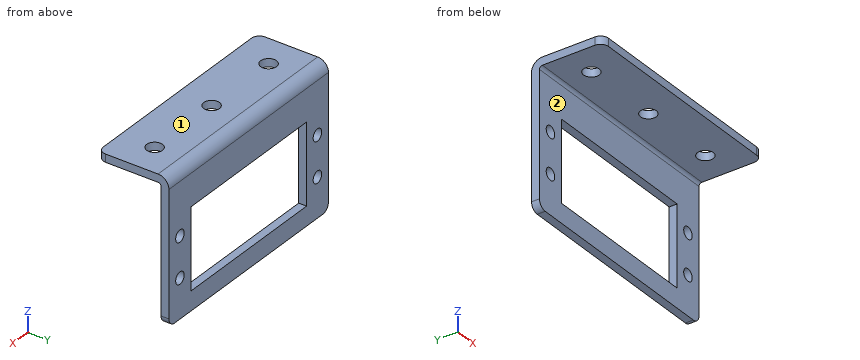
from build123d import *

# Parameters (mm, degrees)
SKETCH1_W                    = 56
SKETCH1_H                    = 34
BASE_FLANGE1_DEPTH           = 2
EDGE_FLANGE1_STRIP_W         = 9.4732
EDGE_FLANGE1_STRIP_H         = 2
EDGE_FLANGE1_STRIP_CUT_DEPTH = 56
EDGE_FLANGE1_DEPTH           = 56
SKETCH9_W                    = 40.64
SKETCH9_H                    = 20.32
CUT_EXTRUDE1_DEPTH           = 39.327535793
SKETCH10_R                   = 1.5
CUT_EXTRUDE2_DEPTH           = 39.327535793
FILLET1_R                    = 2
SKETCH11_R                   = 2
CUT_EXTRUDE3_DEPTH           = 48.581509013


# Sheet-metal steps are written as plain solids
with BuildPart() as part:
    # Sketch1 → Base-Flange1 (new body)
    with BuildSketch(Plane(origin=(0, 0, 0), x_dir=(1, 0, 0), z_dir=(0, 1, 0))):
        Rectangle(SKETCH1_W, SKETCH1_H)
    extrude(amount=-BASE_FLANGE1_DEPTH)

    # Edge-Flange1 strip (across the edge) → Edge-Flange1 strip cut (cut)
    with BuildSketch(Plane(origin=(28, -2, 17), x_dir=(0, 0, -1), z_dir=(-1, 0, 0))):
        with Locations((-4, -1)):
            Rectangle(EDGE_FLANGE1_STRIP_W, EDGE_FLANGE1_STRIP_H)
    extrude(amount=EDGE_FLANGE1_STRIP_CUT_DEPTH, mode=Mode.SUBTRACT)

    # Edge-Flange1 section (across the edge) → Edge-Flange1 (add)
    with BuildSketch(Plane(origin=(28, -2, 17), x_dir=(0, 0, -1), z_dir=(-1, 0, 0))):
        with BuildLine():
            Line((-2, 0.7366), (-2, 16))
            Line((-2, 16), (0, 16))
            Line((0, 16), (0, 0.7366))
            ThreePointArc((0, 0.7366), (0.215745145, 0.215745145), (0.7366, 0))
            Line((0.7366, 0), (0.7366, -2))
            ThreePointArc((0.7366, -2), (-1.198468417, -1.198468417), (-2, 0.7366))
        make_face()
    extrude(amount=EDGE_FLANGE1_DEPTH)

    # Sketch9 → Cut-Extrude1 (cut, through all)
    with BuildSketch(Plane(origin=(0, 0, 0), x_dir=(1, 0, 0), z_dir=(0, 1, 0))):
        with Locations((0, 2)):
            Rectangle(SKETCH9_W, SKETCH9_H)
    extrude(amount=-CUT_EXTRUDE1_DEPTH, mode=Mode.SUBTRACT)

    # Sketch10 → Cut-Extrude2 (cut, through all)
    with BuildSketch(Plane(origin=(0, 0, 0), x_dir=(1, 0, 0), z_dir=(0, 1, 0))):
        with Locations(Location((-24.13, 7.08, 0), (0, 0, 270))):
            Circle(SKETCH10_R)
        with Locations(Location((-24.13, -3.08, 0), (0, 0, 270))):
            Circle(SKETCH10_R)
        with Locations(Location((24.13, 7.08, 0), (0, 0, 270))):
            Circle(SKETCH10_R)
        with Locations(Location((24.13, -3.08, 0), (0, 0, 270))):
            Circle(SKETCH10_R)
    extrude(amount=-CUT_EXTRUDE2_DEPTH, mode=Mode.SUBTRACT)

    # Fillet1
    fillet1_edges = [part.edges().sort_by_distance(p)[0] for p in [
        (28, -18, 18),
        (-28, -18, 18),
        (-28, -1, -17),
        (28, -1, -17),
    ]]
    fillet(fillet1_edges, radius=FILLET1_R)

    # Sketch11 → Cut-Extrude3 (cut, through all)
    with BuildSketch(Plane(origin=(0, 0, 17), x_dir=(-1, 0, 0), z_dir=(0, 0, -1))):
        with Locations(Location((0, -9.3683, 0), (0, 0, 90))):
            Circle(SKETCH11_R)
        with Locations(Location((-20, -9.3683, 0), (0, 0, 90))):
            Circle(SKETCH11_R)
        with Locations(Location((20, -9.3683, 0), (0, 0, 90))):
            Circle(SKETCH11_R)
    extrude(amount=-CUT_EXTRUDE3_DEPTH, mode=Mode.SUBTRACT)


solid = part.part
For this review, take the finished solid that the model builds, in its own axes (mm). Face numbers are marked on the shaded views. A direction names the side the tool comes from. Round coordinates to 2 decimals unless told otherwise and drop trailing zeros. Loops run counter-clockwise (first coordinate to the right, second up) from the corner with the lowest first, then second, coordinate; pieces in that order, holes last. Notation, with made-up numbers: (-18.5, -8) - (30.5, -8) arc R15 ccw to (30.5, 5) - close; hole circle Ø4 at (27.5, 27.5). An arc over 180 degrees is marked (long way). Put each result on its own line as item: value. Start each with the question number.
1. Consider section B-B on z = 3.08. State the section outline as (x, y) points.
2. Consider section D-D on z = -11.5. State the section outline as (x, y) points, plus the area to 3 significant figures.
3. Consider section A-A on x = 10.5. State the section outline as (y, z) points.
4. Consider section C-C on x = -24.13. State the section outline as (y, z) points, plus the area to 3 significant figures.
5. For probe 1 along X at (y, z) = (-0.85, 3.08); probe 2 along Z at (x, y) = (23, -9.5); probe 3 along Y at (x, z) = (22, -0.5), list the stretches that pass through material, from the lowest coordinate up. Write a range as [from, to].
6. For the marked faces 1 and 2, list the 3-axis set-ups (+Z, -Z, +X, -X, +Y, -Y) from which the entire face can be reached by the end or side of a thin tool; tool diameter is ignored.
7. Insertion check: P1, Ø6.5, axis at x = -20, y = -9.37, coming from the -Z side; P2, Ø1, axis at x = -3, z = 11.5, coming from the -Y side; P3, Ø1, axis at x = -9.5, y = -0.5, coming from the +Z side. Each pin has a flat end and moves straight along its axis. Give the tip position at first contact, or say it passes through.
Result sheet:
1. outline: (-28, -2) - (-25.63, -2) - (-25.63, 0) - (-28, 0) - close; (-22.63, -2) - (-20.32, -2) - (-20.32, 0) - (-22.63, 0) - close; (20.32, -2) - (22.63, -2) - (22.63, 0) - (20.32, 0) - close; (25.63, -2) - (28, -2) - (28, 0) - (25.63, 0) - close
2. outline: (-28, -2) - (-20.32, -2) - (-20.32, 0) - (-28, 0) - close; (20.32, -2) - (28, -2) - (28, 0) - (20.32, 0) - close
2. area: 30.7 mm^2
3. outline: (-18, 17) - (-2.74, 17) arc R0.74 cw to (-2, 16.26) - (-2, 8.16) - (0, 8.16) - (0, 16.26) arc R2.74 ccw to (-2.74, 19) - (-18, 19) - close; (-2, -17) - (0, -17) - (0, -12.16) - (-2, -12.16) - close
4. outline: (-18, 17) - (-2.74, 17) arc R0.74 cw to (-2, 16.26) - (-2, 4.58) - (0, 4.58) - (0, 16.26) arc R2.74 ccw to (-2.74, 19) - (-18, 19) - close; (-2, -17) - (0, -17) - (0, -8.58) - (-2, -8.58) - close; (-2, -5.58) - (0, -5.58) - (0, 1.58) - (-2, 1.58) - close
4. area: 90.5 mm^2
5. probe 1: [-28, -25.63], [-22.63, -20.32], [20.32, 22.63], [25.63, 28]
5. probe 2: [17, 19]
5. probe 3: [-2, 0]
6. face 1: +Z, +X, -X, +Y, -Y
6. face 2: -Z, +X, -X, -Y
7. P1: z = 17
7. P2: y = -2
7. P3: z = 18.38
